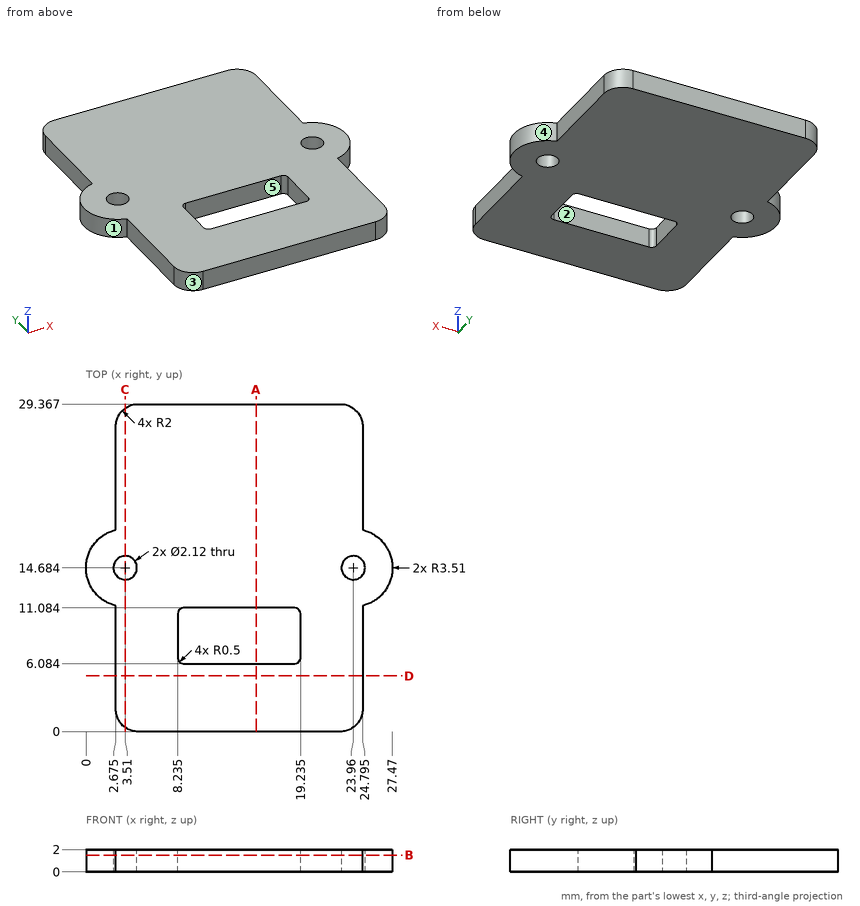
Study the drawing (mm; zero at the part's minimum x, y, z) and answer. A direction names the side the tool comes from. Give positions to 0.01 mm unless a question says otherwise; leave off trailing zeros. Write each loop counter-clockwise with the first axis right and the second up, starting at its lowest first coordinate (ties: lowest second). Pieces come first, ordered by that corner, then holes. Notation, with made-up numbers: M 6,79.25 L 18,79.25 A28 ccw 18,107.25 Z; hole C -16,-31.5 d3. An arc over 180 degrees is marked long. Put each result on its own line as item: value. Start each with the question number.
1. Consider line 1 along Y through (x, z) = (12.25, 1.4); line 2 along X through (y, z) = (27.5, 1.3); line 3 along Y through (x, z) = (23.96, 1.05) (1 decimal). Determine where each line is inside the solid, lowest interval first.
2. For a pull along Y with two mould halves and no side action, classify the marked faces 1, 2 and 3 as released by +Y, released by -Y, zero draft, split by the parting line, or undercut.
3. Which of the six approach directions +Z, -Z, +X, -X, +Y, -Y give full straight-line access (tool end or side, diameter ignored) to the marked faces 4 and 5?
4. Each of these flat-tipped pins is pushed along its axis until it touches: pin 1 Ø3.5 at (x, y) = (23.96, 14.68) entering from -Z; pin 2 Ø0.6 at (y, z) = (21, 1) entering from -X (3 decimals); pin 3 Ø3 at (x, y) = (12, 8) entering from -Z; pin 4 Ø1 at (y, z) = (24.5, 1) entering from +X (3 decimals). Where does it stop, or does it pass through?
5. The part is cut by section B-B, the plane z = 1.5. Give the vertices of the cut face in (x, y) (1 decimal).
6. The part is cut by section A-A, the plane x = 15.25. Give the vertices of the cut face in (y, z).
7. The part is cut by section D-D, the plane y = 5. Give the vertices of the cut face in (x, z) (1 decimal).
8. The part is cut by section C-C, the plane x = 3.51. Give the vertices of the cut face in (y, z) (1 decimal).
Final values:
1. line 1: y = 0 to 6.08, 11.08 to 29.37
1. line 2: x = 2.68 to 24.79
1. line 3: y = 0.4 to 13.6, 15.7 to 29
2. face 1: split by the parting line
2. face 2: undercut
2. face 3: released by -Y
3. face 4: +Z, -Z, +X
3. face 5: +Z, -Z
4. pin 1: stops at z = 0
4. pin 2: stops at x = 2.675
4. pin 3: passes through
4. pin 4: stops at x = 24.795
5. outline: M 2.7,2 A2 ccw 4.7,0 L 22.8,0 A2 ccw 24.8,2 L 24.8,11.3 A3.5 ccw 24.8,18.1 L 24.8,27.4 A2 ccw 22.8,29.4 L 4.7,29.4 A2 ccw 2.7,27.4 L 2.7,18.1 A3.5 ccw 2.7,11.3 Z; hole C 3.5,14.7 d2.1; hole M 8.2,6.6 A0.5 ccw 8.7,6.1 L 18.7,6.1 A0.5 ccw 19.2,6.6 L 19.2,10.6 A0.5 ccw 18.7,11.1 L 8.7,11.1 A0.5 ccw 8.2,10.6 Z; hole C 24,14.7 d2.1
6. outline: M 0,0 L 6.08,0 L 6.08,2 L 0,2 Z; M 11.08,0 L 29.37,0 L 29.37,2 L 11.08,2 Z
7. outline: M 2.7,0 L 24.8,0 L 24.8,2 L 2.7,2 Z
8. outline: M 0.4,0 L 13.6,0 L 13.6,2 L 0.4,2 Z; M 15.7,0 L 29,0 L 29,2 L 15.7,2 Z
